Drawing for the job (mm, zero at the part's lowest x, y, z). A direction names the side the tool comes from. Coordinates: 2 decimals unless noted, no trailing zeros. Write each loop counter-clockwise with the first axis right and the second up, starting at its lowest first coordinate (ties: lowest second). Pieces come first, ordered by that corner, then holes. Notation, with made-up numbers: (-2, 65.5) -> (39, 65.5) arc R5 ccw to (39, 69.5) -> close; hole circle Ø8 at (9.5, -3.5). An arc over 180 degrees is marked (long way). Write each question's results on one line, items separated by ' | '. Start each with the question number.
Q1. Saw through at B-B on x = 7.5. Give the cut face in (y, z), and give its area (3 significant figures).
Q2. Drill centre lines: line 1 (Y direction, x = 21, z = 2.2); line 2 (X direction, y = 9.75, z = 2.7); line 3 (Y direction, x = 41, z = 1.15). Where is each one in solid material? Low to high.
Q3. Tool access for the marked faces 1 and 2: list every direction of +Z, -Z, +X, -X, +Y, -Y with a clear straight run to the whole face (end or side of a thin tool).
Q4. Drop flat-ended pins along their axis: pin 1 Ø1.5 at (y, z) = (2, 1) entering from +X; pin 2 Ø1.5 at (x, z) = (5.5, 0.5) entering from -Y; pin 3 Ø2 at (x, y) = (15.5, 6.5) entering from -Z; pin 4 Ø1.5 at (y, z) = (1.5, 2) entering from -X. Give the stop position or say it passes through.
Q5. Two-plate mould, pull along X, no slides. Class the marked faces 3 and 4: released by +X, released by -X, zero draft, split by the parting line, or undercut.
Q6. Saw through at C-C on y = 4.5. Give the cut face in (x, z).
Q7. Saw through at A-A on z = 1.05. Give the cut face in (x, y), and give its area (3 significant figures).
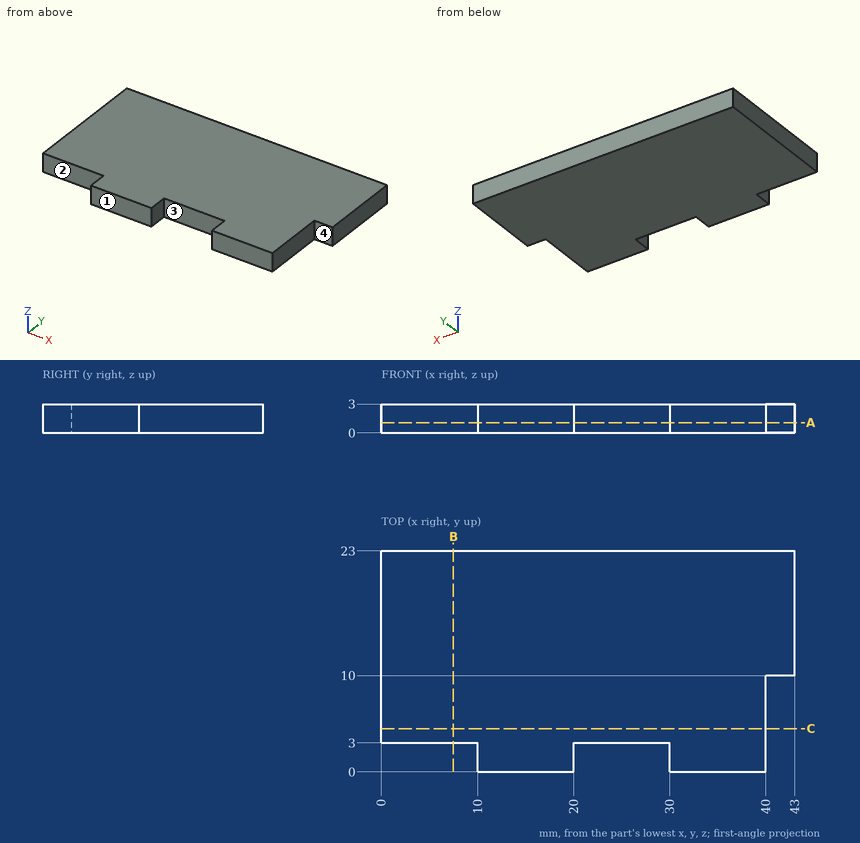
Returned:
1) outline: (3, 0) -> (23, 0) -> (23, 3) -> (3, 3) -> close | area: 60.0 mm2
2) line 1: y = 3 to 23 | line 2: x = 0 to 40 | line 3: y = 10 to 23
3) face 1: +Z, -Z, +X, -X, -Y | face 2: +Z, -Z, -X, -Y
4) pin 1: stops at x = 40 | pin 2: stops at y = 3 | pin 3: stops at z = 0 | pin 4: stops at x = 10
5) face 3: undercut | face 4: zero draft
6) outline: (0, 0) -> (40, 0) -> (40, 3) -> (0, 3) -> close
7) outline: (0, 3) -> (10, 3) -> (10, 0) -> (20, 0) -> (20, 3) -> (30, 3) -> (30, 0) -> (40, 0) -> (40, 10) -> (43, 10) -> (43, 23) -> (0, 23) -> close | area: 899 mm2
